from build123d import *

# Parameters (mm, degrees)
SKETCH1_R           = 2.5
SKETCH1_R_2         = 36.5
BOSS_EXTRUDE1_DEPTH = 4
SKETCH2_R           = 2.5
BOSS_EXTRUDE2_DEPTH = 5
SKETCH3_R           = 64.411178088
CUT_EXTRUDE1_DEPTH  = 10
FILLET1_R           = 5


with BuildPart() as part:
    # Sketch1 → Boss-Extrude1 (new body)
    with BuildSketch(Plane(origin=(0, 0, 0), x_dir=(1, 0, 0), z_dir=(0, 1, 0))):
        with BuildLine():
            ThreePointArc((-35.096538253, 5.994415913), (-29.942413888, -2.588482391), (-39.858946955, -3.964532245))
            ThreePointArc((-39.858946955, -3.964532245), (-41.168529898, -2.983419005), (-42.761405669, -2.608802601))
            ThreePointArc((-42.761405669, -2.608802601), (-52.246827812, -8.771034491), (-49.915694824, -19.839555354))
            ThreePointArc((-49.915694824, -19.839555354), (-49.174030159, -20.398421652), (-48.323482114, -20.771203143))
            ThreePointArc((-48.323482114, -20.771203143), (-31.112698372, -31.112698372), (-20.771203143, -48.323482114))
            ThreePointArc((-20.771203143, -48.323482114), (-20.398421652, -49.174030159), (-19.839555354, -49.915694824))
            ThreePointArc((-19.839555354, -49.915694824), (-8.771034491, -52.246827812), (-2.608802601, -42.761405669))
            ThreePointArc((-2.608802601, -42.761405669), (-2.983419005, -41.168529898), (-3.964532245, -39.858946955))
            ThreePointArc((-3.964532245, -39.858946955), (-2.588482391, -29.942413888), (5.994415913, -35.096538253))
            ThreePointArc((5.994415913, -35.096538253), (6.065284008, -35.692875475), (6.224630915, -36.271882326))
            ThreePointArc((6.224630915, -36.271882326), (3.044943645, -55.463499369), (-14.941352097, -62.87441978))
            ThreePointArc((-14.941352097, -62.87441978), (-17.849646318, -63.67833691), (-19.368850678, -66.285342115))
            ThreePointArc((-19.368850678, -66.285342115), (-89.802561211, -89.802561211), (-66.285342115, -19.368850678))
            ThreePointArc((-66.285342115, -19.368850678), (-63.67833691, -17.849646318), (-62.87441978, -14.941352097))
            ThreePointArc((-62.87441978, -14.941352097), (-55.463499369, 3.044943645), (-36.271882326, 6.224630915))
            ThreePointArc((-36.271882326, 6.224630915), (-35.692875475, 6.065284008), (-35.096538253, 5.994415913))
        make_face()
        with Locations(Location((0, -35.355339059, 0), (0, 0, 270))):
            Circle(SKETCH1_R, mode=Mode.SUBTRACT)
        with Locations(Location((-35.355339059, 0, 0), (0, 0, 270))):
            Circle(SKETCH1_R, mode=Mode.SUBTRACT)
        with Locations(Location((-60.457629791, -60.457629791, 0), (0, 0, 270))):
            Circle(SKETCH1_R_2, mode=Mode.SUBTRACT)
    extrude(amount=BOSS_EXTRUDE1_DEPTH)

    # Sketch2 → Boss-Extrude2 (add)
    # profile 1 of 2: a face of its own
    with BuildSketch(Plane(origin=(0, 4, 0), x_dir=(1, 0, 0), z_dir=(0, 1, 0))):
        Polygon((-32.468587713, -5), (-29.581836367, 0), (-32.468587713, 5), (-38.242090405, 5), (-41.128841751, 0), (-38.242090405, -5), align=None)
        with Locations(Location((-35.355339059, 0, 0), (0, 0, 270))):
            Circle(SKETCH2_R, mode=Mode.SUBTRACT)
    # profile 2 of 2: a face of its own
    with BuildSketch(Plane(origin=(0, 4, 0), x_dir=(1, 0, 0), z_dir=(0, 1, 0))):
        Polygon((-5, -38.242090405), (-5, -32.468587713), (0, -29.581836367), (5, -32.468587713), (5, -38.242090405), (0, -41.128841751), align=None)
        with Locations(Location((0, -35.355339059, 0), (0, 0, 90))):
            Circle(SKETCH2_R, mode=Mode.SUBTRACT)
    extrude(amount=BOSS_EXTRUDE2_DEPTH)

    # Sketch3 → Cut-Extrude1 (cut)
    with BuildSketch(Plane(origin=(0, 4, 0), x_dir=(1, 0, 0), z_dir=(0, 1, 0))):
        with Locations((-87.790328178, -89.76214525)):
            Circle(SKETCH3_R)
    extrude(amount=-CUT_EXTRUDE1_DEPTH, mode=Mode.SUBTRACT)

    # Fillet1
    # the kernel refuses this fillet: 5 mm, written as the material it takes off along each edge
    with BuildSketch(Plane(origin=(-82.88269404, 36.492109743, 25.538201196), x_dir=(0.9156666742355372, 0, -0.40193847998721216), z_dir=(0, -1, 0))) as fillet1_piece_1:
        with BuildLine():
            CenterArc((12.213901494, 4.938319673), FILLET1_R, 185.081491193, 93.927443362)
            ThreePointArc((7.233552845, 4.495457015), (3.691158281, 2.128042099), (0, 0))
            ThreePointArc((0, 0), (6.498421949, -0.511946714), (12.996843897, 0))
        make_face()
    extrude(amount=68.984219486, mode=Mode.SUBTRACT)
    with BuildSketch(Plane(origin=(-24.063187691, 36.492109743, 80.399911111), x_dir=(-0.2104426135040135, 0, -0.9776062123481011), z_dir=(0, -1, 0))) as fillet1_piece_2:
        with BuildLine():
            CenterArc((12.98043651, 2.252700357), FILLET1_R, 112.850896292, 93.927443362)
            ThreePointArc((11.038764851, 6.860293131), (5.249154934, 3.86496439), (0, 0))
            ThreePointArc((0, 0), (4.258327739, 0.140916633), (8.516655478, 0))
        make_face()
    extrude(amount=68.984219486, mode=Mode.SUBTRACT)


solid = part.part
Source: CAD feature listing. Evaluate the final solid. Frame: model axes, mm. A direction names the side the tool comes from. Round coordinates to 2 decimals unless told otherwise and drop trailing zeros. Loops run counter-clockwise (first coordinate to the right, second up) from the corner with the lowest first, then second, coordinate; pieces in that order, holes last. Notation, with made-up numbers: M -21,53 L 27,53 A27 cw 27,80 Z; hole C -16.5,-30.75 d4. An arc over 180 degrees is marked long. Answer as CSV lines item,"result".
Q1. Cut plane D-D (y = 1.5). Return the cut outline in (x, z), plus the area to 3 significant figures.
Verdict:
outline,"M -74.45,26.75 A5 ccw -70.98,20.31 A41.5 ccw -66.29,19.37 A4 cw -62.87,14.94 A20 ccw -36.27,-6.22 A4 cw -35.1,-5.99 A6 ccw long -39.86,3.96 A4 cw -42.76,2.61 A10 cw -49.92,19.84 A4 cw -48.32,20.77 A41.5 ccw -20.77,48.32 A4 cw -19.84,49.92 A10 cw -2.61,42.76 A4 cw -3.96,39.86 A6 ccw long 5.99,35.1 A4 cw 6.22,36.27 A20 ccw -14.94,62.87 A4 cw -19.37,66.29 A41.5 ccw -19.68,68.16 A5 ccw -25.86,72.07 A36.5 cw Z; hole C -35.36,0 d5; hole C 0,35.36 d5"
area,"1,300 mm^2"
Q2. Line query: line 1 along X through (y, z) = (4.5, 0); line 2 along Y through (x, z) = (-6, 59); line 3 along X through (y, z) = (2.75, 0). Output: solid intervals per line, ascending.
Verdict:
line 1,"x = -41.13 to -37.86, -32.86 to -29.58"
line 2,"y = 0 to 4"
line 3,"x = -58.54 to -37.86, -32.86 to -29.36"
Q3. Contact query for flat-ended pins moving along their axis: pin 1 (4 mm diameter, centred on x = 0, z = 35.36, fed in from +Y); pin 2 (1.5 mm diameter, centred on x = -36.5, y = 6, fed in from +Z); pin 3 (4 mm diameter, centred on y = 4.5, z = 51.5, fed in from +X); pin 4 (2.5 mm diameter, centred on y = 7.5, z = 36, fed in from +X). Output: stop coordinate, or through.
Verdict:
pin 1,"passes through"
pin 2,"stops at z = 5"
pin 3,"stops at x = 6.29"
pin 4,"stops at x = 5"
Q4. Cut plane C-C (x = -46.5). Return the cut outline in (y, z).
Verdict:
outline,"M 0,-7.09 L 4,-7.09 L 4,3.23 L 0,3.23 Z; M 0,21.38 L 4,21.38 L 4,26.73 L 0,26.73 Z"
Q5. Cut plane A-A (y = 5.75). Return the cut outline in (x, z).
Verdict:
outline,"M -41.13,0 L -38.24,-5 L -32.47,-5 L -29.58,0 L -32.47,5 L -38.24,5 Z; M -5,32.47 L 0,29.58 L 5,32.47 L 5,38.24 L 0,41.13 L -5,38.24 Z; hole C -35.36,0 d5; hole C 0,35.36 d5"
Q6. Cut plane B-B (z = 46). Return the cut outline in (x, y).
Verdict:
outline,"M -26.94,0 L -21.56,0 L -21.56,4 L -26.94,4 Z; M -3.06,0 L 7.17,0 L 7.17,4 L -3.06,4 Z"
Q7. Pull-direction query (X, two-part tool) for faces 6 (the face through (-35, 6, -5)), 7 (the face through (-29.873, 1.972, 2.438)), 8 (the face through (-19.51, 1.97, 67.21)); classes: +X half, -X half, draft (parallel to the pull), parting line (faces both ways), or undercut.
Verdict:
face 6,"draft"
face 7,"undercut"
face 8,"+X half"
Q8. Reachability of faces 1 (the face through (2.53, 6.46, 39.67)), 2 (the face through (-31.01, 6.46, -2.47)), 3 (the face through (-2.535, 6.465, 31.045)), 4 (the face through (-52.181, 1.972, 8.616)), 5 (the face through (-5, 6, 35)) from +Z, -Z, +X, -X, +Y, -Y: full face, straight path, thin tool, end or side. Return the list, or none.
Verdict:
face 1,"+Z, +X, +Y"
face 2,"-Z, +X, +Y"
face 3,"-Z, -X, +Y"
face 4,"+Y, -Y"
face 5,"+Z, -Z, -X, +Y"
